```python
from build123d import *

# Parameters (mm, degrees)
SKETCH1_W               = 150
SKETCH1_H               = 97
BOSS_EXTRUDE2_DEPTH     = 64
CUT_EXTRUDE1_DEPTH      = 190.74983531
CUT_EXTRUDE1_DEPTH_BACK = 9
SKETCH4_R               = 3.5
SKETCH4_W               = 15
SKETCH4_H               = 7
SKETCH4_W_2             = 1
SKETCH4_H_2             = 8
CUT_EXTRUDE2_DEPTH      = 2


with BuildPart() as part:
    # Sketch1 → Boss-Extrude2 (new body)
    with BuildSketch(Plane.XY):
        with Locations((75, -48.5)):
            Rectangle(SKETCH1_W, SKETCH1_H)
    extrude(amount=BOSS_EXTRUDE2_DEPTH)

    # Sketch3 → Cut-Extrude1 (cut, two sides: drawn at the far end of the back side and taken through both)
    with BuildSketch(Plane(origin=(0, 0, 0), x_dir=(1, 0, 0), z_dir=(0, 1, 0)).offset(-CUT_EXTRUDE1_DEPTH_BACK)):
        Polygon((20, 299.799930987), (20, 0), (20, -1), (149, -1), (149, -63), (20, -63), (20, -64), (20, -363.799930987), (619.599861974, -363.799930987), (619.599861974, 299.799930987), align=None)
    extrude(amount=CUT_EXTRUDE1_DEPTH + CUT_EXTRUDE1_DEPTH_BACK, mode=Mode.SUBTRACT)

    # Sketch4 → Cut-Extrude2 (cut)
    with BuildSketch(Plane(origin=(0, 0, 0), x_dir=(1, 0, 0), z_dir=(0, 1, 0))):
        with Locations(Location((7, -32, 0), (0, 0, 270))):
            Circle(SKETCH4_R)
        with Locations((10.5, -8.5)):
            Rectangle(SKETCH4_W, SKETCH4_H)
        with Locations((10.5, -55.5)):
            Rectangle(SKETCH4_W, SKETCH4_H)
        Polygon((6.5, -16), (6.5, -19.5), (3, -19.5), (3, -20.5), (6.5, -20.5), (6.5, -24), (7.5, -24), (7.5, -20.5), (11, -20.5), (11, -19.5), (7.5, -19.5), (7.5, -16), align=None)
        with Locations((7, -44)):
            Rectangle(SKETCH4_W_2, SKETCH4_H_2)
    extrude(amount=-CUT_EXTRUDE2_DEPTH, mode=Mode.SUBTRACT)


solid = part.part
```
Model file for the job. Use its own axes, mm. A direction names the side the tool comes from. Coordinates: 2 decimals unless noted, no trailing zeros. Answer as a JSON object with one key per item and string values.
Q1. Pull direction Z, two halves, no side cores. Call faces 1 (the flat face through (74, -48, 64)), 2 (the flat face through (73, 0, 32)), 3 (the flat face through (10, -2, 8)), 4 (the flat face through (7, -2, 20)): released by +Z, released by -Z, zero draft, split by the parting line, or undercut.
Report:
{"face 1": "released by +Z", "face 2": "zero draft", "face 3": "undercut", "face 4": "undercut"}
Q2. Flat gauge pins, fed straight in: P1, Ø0.6, axis at y = -1, z = 57, coming from the +X side; P2, Ø0.5, axis at x = 7, z = 44.5, coming from the +Y side; P3, Ø4.5, axis at x = 54, y = -3.5, coming from the -Z side. Where does each tip first touch, or does it go through?
Report:
{"P1": "stops at x = 149", "P2": "stops at y = -2", "P3": "stops at z = 1"}
Q3. 3-axis set-ups, long thin cutter, end or side, ignore diameter. For faces 5 (the flat face through (85, -5, 63)), 6 (the flat face through (10, -2, 55)), 7 (the flat face through (84, -5, 1)): which of +Z, -Z, +X, -X, +Y, -Y reach the whole face in a straight line?
Report:
{"face 5": "+Z, +X, +Y", "face 6": "+Y", "face 7": "-Z, +X, +Y"}
Q4. Probe probe 1 along X at (y, z) = (-1.1, 32). List the from-to ranges inside material, lowest first.
Report:
{"probe 1": "x = 0 to 3.5, 10.5 to 149"}
